Can you work these out from the model? Positions are in its coordinate system, mm. A direction names the side the tool comes from. Give positions to 0.01 mm unless a question says otherwise; leave off trailing zeros. Order: outer loops, then holes, each group sorted by start corner. A loop starts at its lowest first (then second) coordinate and runs counter-clockwise, first axis right, second up. Notation, with made-up numbers: (-33, -22) - (21, -22) arc R18 cw to (21, -3) - close; hole circle Ø9 at (29, -28). An arc over 180 degrees is marked (long way). Return JSON: item names as keys, results as strings.
```python
from build123d import *

# Parameters (mm, degrees)
EXTRUDE_1_DEPTH     = 25
SKETCH_2_R          = 2.1
CUT_EXTRUDE_1_DEPTH = 25
SKETCH_4_R          = 4
CUT_EXTRUDE_2_DEPTH = 24
SKETCH_5_R          = 2.044965575
CUT_EXTRUDE_3_DEPTH = 24
SKETCH_6_R          = 4
CUT_EXTRUDE_4_DEPTH = 30.5


with BuildPart() as part:
    # 草圖1 → 填料-伸長1 (new body)
    with BuildSketch(Plane.XY):
        with BuildLine():
            Line((-3.252259835, 16.056494785), (-32.252259835, 16.056494785))
            Line((-32.252259835, 16.056494785), (-32.252259835, 11.056494785))
            add(Edge.make_bspline(
                [(-8.252259835, -19.443505215), (-8.252259835, 11.056494785), (-32.252259835, 11.056494785)],
                knots=[4.71238898, 4.71238898, 4.71238898, 6.283185307, 6.283185307, 6.283185307], degree=2, weights=[1, 0.707106781, 1]))
            Line((-8.252259835, -19.443505215), (-3.252259835, -19.443505215))
            Line((-3.252259835, -19.443505215), (-3.252259835, 16.056494785))
        make_face()
    extrude(amount=EXTRUDE_1_DEPTH)

    # 草圖2 → 除料-伸長1 (cut)
    with BuildSketch(Plane(origin=(-3.252259835, 0, 0), x_dir=(0, 0, -1), z_dir=(1, 0, 0))):
        with Locations(Location((-20, -14.443505215, 0), (0, 0, 90))):
            Circle(SKETCH_2_R)
        with Locations(Location((-5, -14.443505215, 0), (0, 0, 90))):
            Circle(SKETCH_2_R)
        with Locations(Location((-5, -5.443505215, 0), (0, 0, 90))):
            Circle(SKETCH_2_R)
        with Locations(Location((-5, 3.556494785, 0), (0, 0, 90))):
            Circle(SKETCH_2_R)
        with Locations(Location((-20, -5.443505215, 0), (0, 0, 90))):
            Circle(SKETCH_2_R)
        with Locations(Location((-20, 3.556494785, 0), (0, 0, 90))):
            Circle(SKETCH_2_R)
    extrude(amount=-CUT_EXTRUDE_1_DEPTH, mode=Mode.SUBTRACT)

    # 草圖4 → 除料-伸長2 (cut)
    with BuildSketch(Plane.ZY.offset(32.252259835)):
        with Locations((5, 3.556494785)):
            Circle(SKETCH_4_R)
        with Locations((20, 3.556494785)):
            Circle(SKETCH_4_R)
        with Locations((20, -5.443505215)):
            Circle(SKETCH_4_R)
        with Locations((20, -14.443505215)):
            Circle(SKETCH_4_R)
        with Locations((5, -5.443505215)):
            Circle(SKETCH_4_R)
        with Locations((5, -14.443505215)):
            Circle(SKETCH_4_R)
    extrude(amount=-CUT_EXTRUDE_2_DEPTH, mode=Mode.SUBTRACT)

    # 草圖5 → 除料-伸長3 (cut)
    with BuildSketch(Plane(origin=(0, 16.056494785, 0), x_dir=(1, 0, 0), z_dir=(0, 1, 0))):
        with Locations(Location((-27.252259835, -5, 0), (0, 0, 270))):
            Circle(SKETCH_5_R)
        with Locations(Location((-27.252259835, -20, 0), (0, 0, 270))):
            Circle(SKETCH_5_R)
    extrude(amount=-CUT_EXTRUDE_3_DEPTH, mode=Mode.SUBTRACT)

    # 草圖6 → 除料-伸長4 (cut)
    with BuildSketch(Plane.XZ.offset(19.443505215)):
        with Locations(Location((-27.252259835, 5, 0), (0, 0, 270))):
            Circle(SKETCH_6_R)
        with Locations(Location((-27.252259835, 20, 0), (0, 0, 270))):
            Circle(SKETCH_6_R)
    extrude(amount=-CUT_EXTRUDE_4_DEPTH, mode=Mode.SUBTRACT)


solid = part.part
```
1. Thinking about a two-plate mould opening in Z: for faces 4 (the face through (-23.286, 10.175, 5.521)), 5 (the face through (-12, 2, 25)), 6 (the face through (-32.252, 14, 12)), which applies, +Z half, -Z half, draft (parallel to the pull), parting line (faces both ways), or undercut?
Checks:
{"face 4": "undercut", "face 5": "+Z half", "face 6": "draft"}
2. On a 3-axis mill with a long thin cutter (end or side, diameter ignored), from which of +Z, -Z, +X, -X, +Y, -Y can I reach the whole of each face in a straight line? I mean faces 1 (the face through (-26, 11.056, 22)), 2 (the face through (-5.72, 3.28, 7.08)), 3 (the face through (-8.252, -16, 7)). Say none if no direction works.
Checks:
{"face 1": "-Y", "face 2": "+X, -X", "face 3": "-X"}
3. For pin 1 Ø3 at (x, z) = (-24.5, 4) entering from -Y; pin 2 Ø4 at (y, z) = (-6, 6) entering from -X; pin 3 Ø13 at (y, z) = (3.56, 20) entering from -X, each with a flat end and sliding along its axis, tell me the tip position at first contact or that it passes through.
Checks:
{"pin 1": "y = 8.7", "pin 2": "x = -8.25", "pin 3": "x = -24.45"}
4. Suppose I cut it at A-A (x = -5.5). List the corners of the cut face in (y, z) for me.
Checks:
{"outline": "(-19.44, 0) - (16.06, 0) - (16.06, 25) - (-19.44, 25) - close; hole circle Ø4.2 at (-14.44, 5); hole circle Ø4.2 at (-14.44, 20); hole circle Ø4.2 at (-5.44, 5); hole circle Ø4.2 at (-5.44, 20); hole circle Ø4.2 at (3.56, 5); hole circle Ø4.2 at (3.56, 20)"}
5. If I drill on L1, parallel to Y at x = -9.1, z = 20; L2, parallel to X at y = -4, z = 2.5; L3, parallel to Z at x = -7, y = -4.5, over which ranges is the centre line in solid material (lowest first)? Write a range as [from, to].
Checks:
{"L1": "[-10.44, -9.44], [-1.44, -0.44], [7.56, 16.06]", "L2": "[-8.25, -3.25]", "L3": "[0, 3.12], [6.88, 18.12], [21.88, 25]"}
6. Suppose I cut it at B-B (z = 20). State how many separate pieces and enclosed holes the cut face has, plus the area to 3 significant figures.
Checks:
{"separate pieces": "5", "enclosed holes": "0", "area": "271 mm^2"}
